For this review, take the finished solid that the model builds, in its own axes (mm). Round coordinates to 2 decimals unless told otherwise and drop trailing zeros. Loops run counter-clockwise (first coordinate to the right, second up) from the corner with the lowest first, then second, coordinate; pieces in that order, holes last.
1) Take a section at C-C (z = 0.6). Give the number of separate pieces and of enclosed holes in the cut face, then the cut area to 3 significant figures.
2) Take a section at D-D (y = 272.5). State the section outline as (x, z) points, then the cut area to 3 significant figures.
3) Take a section at A-A (y = 155). State the section outline as (x, z) points.
4) Take a section at B-B (x = 90). State the section outline as (y, z) points, then the cut area to 3 significant figures.
5) Insertion check: pin 1 (1.5 mm diameter, centred on x = 109, z = 2.5, fed in from +Y); pin 2 (0.9 mm diameter, centred on x = 135, z = 1.5, fed in from +Y); pin 3 (0.9 mm diameter, centred on y = 216, z = 1, fed in from -X). Each pin has a flat end and moves straight along its axis. Give the tip position at first contact, or say it passes through.
6) Wall thickness on L1, parallel to X at y = 266, z = 1.95; L2, parallel to X at y = 243.5, z = 2.2; L3, parallel to X at y = 155.5, z = 2.15: over which ranges is each line inside the solid? List them lowest first.
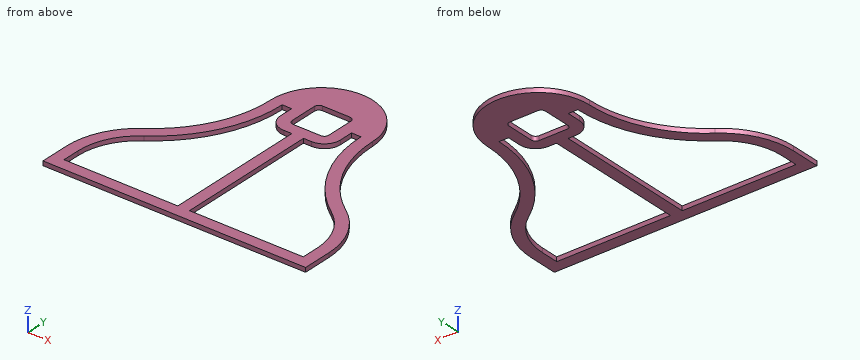
```python
from build123d import *

# Parameters (mm, degrees)
ESQUISSE1_W                  = 180
ESQUISSE1_H                  = 300
BOSS_EXTRU_1_DEPTH           = 15
ESQUISSE2_W                  = 180
ESQUISSE2_H                  = 8.1
ENL_V_MAT_EXTRU_1_DEPTH      = 5
ENL_V_MAT_EXTRU_2_DEPTH      = 10
ENL_V_START                  = -180
ENL_V_MAT_EXTRU_3_DEPTH      = 10
ENL_V_MAT_EXTRU_4_DEPTH      = 351.178525898
ENL_V_MAT_EXTRU_4_DEPTH_BACK = 351.178525898
CONG_1_R                     = 50
ENL_V_MAT_EXTRU_5_DEPTH      = 351.178525898
ENL_V_MAT_EXTRU_5_DEPTH_BACK = 351.178525898
ESQUISSE5_W                  = 25
ESQUISSE5_H                  = 25
CONG_2_R                     = 3
ENL_V_MAT_EXTRU_6_DEPTH      = 351.178525898
ENL_V_MAT_EXTRU_6_DEPTH_BACK = 351.178525898
ESQUISSE6_W                  = 180
ESQUISSE6_H                  = 138.816197092
ENL_V_MAT_EXTRU_7_DEPTH      = 12
ENL_V_MAT_EXTRU_8_DEPTH      = 350.869975848
ENL_V_MAT_EXTRU_8_DEPTH_BACK = 350.869975848
ESQUISSE10_W                 = 8
ESQUISSE10_H                 = 97.683802908
BOSS_EXTRU_2_DEPTH           = 3


with BuildPart() as part:
    # Esquisse1 → Boss.-Extru.1 (new body)
    with BuildSketch(Plane.XY):
        with Locations((90, 150)):
            Rectangle(ESQUISSE1_W, ESQUISSE1_H)
    extrude(amount=BOSS_EXTRU_1_DEPTH)

    # Esquisse2 → Enlèv. mat.-Extru.1 (cut)
    with BuildSketch(Plane.XY.offset(15)):
        with Locations((90, 12.05)):
            Rectangle(ESQUISSE2_W, ESQUISSE2_H)
    extrude(amount=-ENL_V_MAT_EXTRU_1_DEPTH, mode=Mode.SUBTRACT)

    # Esquisse3 → Enlèv. mat.-Extru.2 (cut)
    with BuildSketch(Plane.ZY):
        Polygon((0, 35), (0, 5), (15, 7.644904711), (15, 32.355095289), align=None)
        Polygon((0, 51), (15, 53.644904711), (15, 78.355095289), (0, 81), align=None)
    extrude(amount=-ENL_V_MAT_EXTRU_2_DEPTH, mode=Mode.SUBTRACT)

    # Esquisse3<2> → Enlèv. mat.-Extru.3 (cut)
    with BuildSketch(Plane.ZY.offset(ENL_V_START)):
        Polygon((0, 35), (0, 5), (15, 7.644904711), (15, 32.355095289), align=None)
        Polygon((0, 51), (15, 53.644904711), (15, 78.355095289), (0, 81), align=None)
    extrude(amount=ENL_V_MAT_EXTRU_3_DEPTH, mode=Mode.SUBTRACT)

    # Esquisse4 → Enlèv. mat.-Extru.4 (cut, two sides: drawn at the far end of the back side and taken through both)
    with BuildSketch(Plane(origin=(0, 0, 0), x_dir=(-1, 0, 0), z_dir=(0, 0, -1)).offset(-ENL_V_MAT_EXTRU_4_DEPTH_BACK)):
        with BuildLine():
            Line((0, 189.006579232), (0, 300))
            Line((0, 300), (-90, 310))
            Line((-90, 310), (-180, 300))
            Line((-180, 300), (-180, 189.006579232))
            ThreePointArc((-180, 189.006579232), (-140.192593016, 218.095842402), (-125, 265))
            ThreePointArc((-125, 265), (-90, 300), (-55, 265))
            ThreePointArc((-55, 265), (-39.807406984, 218.095842402), (0, 189.006579232))
        make_face()
    extrude(amount=ENL_V_MAT_EXTRU_4_DEPTH + ENL_V_MAT_EXTRU_4_DEPTH_BACK, mode=Mode.SUBTRACT)

    # Congé1
    cong_1_edges = [part.edges().sort_by_distance(p)[0] for p in [
        (0, 189.006579232, 7.5),
        (180, 189.006579232, 7.5),
    ]]
    fillet(cong_1_edges, radius=CONG_1_R)

    # Esquisse5 → Enlèv. mat.-Extru.5 (cut, two sides: drawn at the far end of the back side and taken through both)
    with BuildSketch(Plane(origin=(0, 0, 0), x_dir=(-1, 0, 0), z_dir=(0, 0, -1)).offset(-ENL_V_MAT_EXTRU_5_DEPTH_BACK)):
        with Locations((-90, 265)):
            Rectangle(ESQUISSE5_W, ESQUISSE5_H)
    extrude(amount=ENL_V_MAT_EXTRU_5_DEPTH + ENL_V_MAT_EXTRU_5_DEPTH_BACK, mode=Mode.SUBTRACT)

    # Congé2
    cong_2_edges = [part.edges().sort_by_distance(p)[0] for p in [
        (77.5, 277.5, 7.5),
        (77.5, 252.5, 7.5),
        (102.5, 252.5, 7.5),
        (102.5, 277.5, 7.5),
    ]]
    fillet(cong_2_edges, radius=CONG_2_R)

    # Esquisse6 → Enlèv. mat.-Extru.6 (cut, two sides: drawn at the far end of the back side and taken through both)
    with BuildSketch(Plane.XY.offset(15).offset(-ENL_V_MAT_EXTRU_6_DEPTH_BACK)):
        with Locations((90, 69.408098546)):
            Rectangle(ESQUISSE6_W, ESQUISSE6_H)
    extrude(amount=ENL_V_MAT_EXTRU_6_DEPTH + ENL_V_MAT_EXTRU_6_DEPTH_BACK, mode=Mode.SUBTRACT)

    # Esquisse8 → Enlèv. mat.-Extru.7 (cut)
    with BuildSketch(Plane.XY.offset(15)):
        with BuildLine():
            Line((0, 158.816197092), (0, 138.816197092))
            Line((0, 138.816197092), (180, 138.816197092))
            Line((180, 138.816197092), (180, 158.816197092))
            ThreePointArc((180, 158.816197092), (174.397678387, 181.812852367), (158.846153846, 199.656121287))
            ThreePointArc((158.846153846, 199.656121287), (133.963714581, 228.20535156), (125, 265))
            ThreePointArc((125, 265), (90, 300), (55, 265))
            ThreePointArc((55, 265), (46.036285419, 228.20535156), (21.153846154, 199.656121287))
            ThreePointArc((21.153846154, 199.656121287), (5.602321613, 181.812852367), (0, 158.816197092))
        make_face()
        with BuildLine():
            Line((102.5, 274.5), (102.5, 255.5))
            ThreePointArc((102.5, 255.5), (101.621320344, 253.378679656), (99.5, 252.5))
            Line((99.5, 252.5), (80.5, 252.5))
            ThreePointArc((80.5, 252.5), (78.378679656, 253.378679656), (77.5, 255.5))
            Line((77.5, 255.5), (77.5, 274.5))
            ThreePointArc((77.5, 274.5), (78.378679656, 276.621320344), (80.5, 277.5))
            Line((80.5, 277.5), (99.5, 277.5))
            ThreePointArc((99.5, 277.5), (101.621320344, 276.621320344), (102.5, 274.5))
        make_face(mode=Mode.SUBTRACT)
    extrude(amount=-ENL_V_MAT_EXTRU_7_DEPTH, mode=Mode.SUBTRACT)

    # Esquisse9 → Enlèv. mat.-Extru.8 (cut, two sides: drawn at the far end of the back side and taken through both)
    with BuildSketch(Plane.XY.offset(3).offset(-ENL_V_MAT_EXTRU_8_DEPTH_BACK)):
        with BuildLine():
            Line((110.5, 255.5), (110.5, 265))
            Line((110.5, 265), (117, 265))
            ThreePointArc((117, 265), (126.860086039, 224.525886716), (154.230769231, 193.121733416))
            ThreePointArc((154.230769231, 193.121733416), (167.294049845, 178.133387523), (172, 158.816197092))
            Line((172, 158.816197092), (172, 146.816197092))
            Line((172, 146.816197092), (8, 146.816197092))
            Line((8, 146.816197092), (8, 158.816197092))
            ThreePointArc((8, 158.816197092), (12.705950155, 178.133387523), (25.769230769, 193.121733416))
            ThreePointArc((25.769230769, 193.121733416), (53.139913961, 224.525886716), (63, 265))
            Line((63, 265), (69.5, 265))
            Line((69.5, 265), (69.5, 255.5))
            ThreePointArc((69.5, 255.5), (72.721825407, 247.721825407), (80.5, 244.5))
            Line((80.5, 244.5), (99.5, 244.5))
            ThreePointArc((99.5, 244.5), (107.278174593, 247.721825407), (110.5, 255.5))
        make_face()
    extrude(amount=ENL_V_MAT_EXTRU_8_DEPTH + ENL_V_MAT_EXTRU_8_DEPTH_BACK, mode=Mode.SUBTRACT)

    # Esquisse10 → Boss.-Extru.2 (add)
    with BuildSketch(Plane.XY.offset(3)):
        with Locations((90, 195.658098546)):
            Rectangle(ESQUISSE10_W, ESQUISSE10_H)
    extrude(amount=-BOSS_EXTRU_2_DEPTH)


solid = part.part
```
Response:
1. separate pieces: 1
1. enclosed holes: 3
1. area: 6,500 mm2
2. outline: (55.81, 0) - (77.5, 0) - (77.5, 3) - (55.81, 3) - close; (102.5, 0) - (124.19, 0) - (124.19, 3) - (102.5, 3) - close
2. area: 130 mm2
3. outline: (0, 0) - (8, 0) - (8, 3) - (0, 3) - close; (86, 0) - (94, 0) - (94, 3) - (86, 3) - close; (172, 0) - (180, 0) - (180, 3) - (172, 3) - close
4. outline: (138.82, 0) - (252.5, 0) - (252.5, 3) - (138.82, 3) - close; (277.5, 0) - (300, 0) - (300, 3) - (277.5, 3) - close
4. area: 409 mm2
5. pin 1: stops at y = 294.87
5. pin 2: stops at y = 227.09
5. pin 3: stops at x = 37.89
6. L1: x = 55.01 to 77.5, 102.5 to 124.99
6. L2: x = 52.06 to 60.33, 86 to 94, 119.67 to 127.94
6. L3: x = 0 to 8, 86 to 94, 172 to 180
